```python
from build123d import *

# Parameters (mm, degrees)
F0_W     = 6.35
F0_H     = 3.175
F3_DEPTH = 50.8
F5_DEPTH = 50.8


with BuildPart() as f1:
    # F0 (on Top) → F1 (revolve)
    with BuildSketch(Plane.XY):
        with Locations((3.175, 39.6875)):
            Rectangle(F0_W, F0_H)
        Polygon((6.35, 38.1), (0, 38.1), (0, -38.1), (6.35, -38.1), (12.7, -38.1), (12.7, 38.1), align=None)
        with Locations((3.175, -39.6875)):
            Rectangle(F0_W, F0_H)
    revolve(axis=Axis((0, 0, 0), (0, -1, 0)))

    # F2 (on face) → F3 (join)
    with BuildSketch(Plane(origin=(0, 41.275, 0), x_dir=(-1, 0, 0), z_dir=(0, 1, 0))):
        Polygon((7.332348, 0), (3.666174, 6.35), (-3.666174, 6.35), (-7.332348, 0), (-3.666174, -6.35), (3.666174, -6.35), align=None)
    extrude(amount=F3_DEPTH)

    # F4 (on face) → F5 (join)
    with BuildSketch(Plane.XZ.offset(41.275)):
        Polygon((7.332348, 0), (3.666174, 6.35), (-3.666174, 6.35), (-7.332348, 0), (-3.666174, -6.35), (3.666174, -6.35), align=None)
    extrude(amount=F5_DEPTH)


solid = f1.part
```
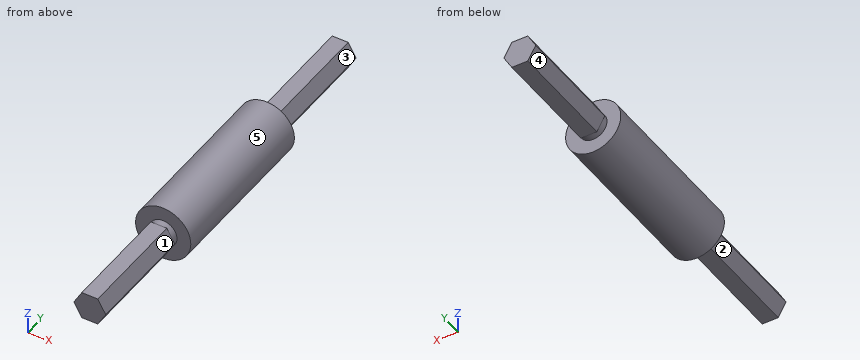
CAD build for the part. Positions are in the model's coordinates, mm. Face numbers are marked on the shaded views. A direction names the side the tool comes from. Round coordinates to 2 decimals unless told otherwise and drop trailing zeros. Loops run counter-clockwise (first coordinate to the right, second up) from the corner with the lowest first, then second, coordinate; pieces in that order, holes last. Notation, with made-up numbers: M 54.5,7 L 95.5,7 A25 ccw 95.5,24 Z; hole C 44.5,70.25 d2. An arc over 180 degrees is marked long. Use a Markdown table: item, result. Add a question column.
(1) Cut at C-C (x = -11). Give the cut face in (y, z).
(2) Flat gauge pins, fed straight in: pin 1 (6 mm diameter, centred on x = 0.5, y = -68, fed in from -Z); pin 2 (4 mm diameter, centred on y = -45.5, z = 8, fed in from +X); pin 3 (1 mm diameter, centred on x = -9.5, z = 2, fed in from +Y). Where does each tip first touch, or does it go through?
(3) Drill centre lines: line 1 (Y direction, x = 3.25, z = 5.75) (3 decimals); line 2 (Z direction, x = 0.25, y = -66.5); line 3 (Z direction, x = 0.5, y = -26). Where is each one in solid material? Low to high.
(4) Which spindle directions (+Z, -Z, +X, -X, +Y, -Y) get a long thin tool onto all of the face, cutting with end or side? Do the marked faces 1, 2, 3, 4 and 5. Say none if no direction does.
(5) Cut at A-A (x = 1.75). Give the cut face in (y, z) (3 decimals).
(6) Cut at B-B (y = 11.5). Give the cut face in (x, z).
Geometry says:
| question | item | result |
|---|---|---|
| 1 | outline | M -38.1,-6.35 L 38.1,-6.35 L 38.1,6.35 L -38.1,6.35 Z |
| 2 | pin 1 | stops at z = -6.35 |
| 2 | pin 2 | stops at x = 3.87 |
| 2 | pin 3 | stops at y = 38.1 |
| 3 | line 1 | y = -92.075 to -41.275, -38.1 to 38.1, 41.275 to 92.075 |
| 3 | line 2 | z = -6.35 to 6.35 |
| 3 | line 3 | z = -12.69 to 12.69 |
| 4 | face 1 | +Z, +X, -Y |
| 4 | face 2 | -Z, -X, -Y |
| 4 | face 3 | +Z, +X, +Y |
| 4 | face 4 | -Z, -X, +Y |
| 4 | face 5 | +Y, -Y |
| 5 | outline | M -92.075,-6.35 L -41.275,-6.35 L -41.275,-6.104 L -38.1,-6.104 L -38.1,-12.579 L 38.1,-12.579 L 38.1,-6.104 L 41.275,-6.104 L 41.275,-6.35 L 92.075,-6.35 L 92.075,6.35 L 41.275,6.35 L 41.275,6.104 L 38.1,6.104 L 38.1,12.579 L -38.1,12.579 L -38.1,6.104 L -41.275,6.104 L -41.275,6.35 L -92.075,6.35 Z |
| 6 | outline | C 0,0 d25.4 |
